Source: CAD feature listing. Evaluate the final solid. Frame: model axes, mm. A direction names the side the tool comes from. Round coordinates to 2 decimals unless told otherwise and drop trailing zeros. Loops run counter-clockwise (first coordinate to the right, second up) from the corner with the lowest first, then second, coordinate; pieces in that order, holes last. Notation, with made-up numbers: (72, 66) - (107, 66) arc R27 cw to (107, 91) - close; hole circle Ø1 at (53, 32.25). An arc over 180 degrees is marked (long way). Write item = value, one per line. Start each with the question number.
from build123d import *

# Parameters (mm, degrees)
SKETCH_W        = 40
SKETCH_H        = 40
PAD_DEPTH       = 5
SKETCH001_W     = 40
SKETCH001_H     = 5
PAD001_DEPTH    = 71
PAD002_DEPTH    = 40
SKETCH004_R     = 2.1
POCKET_DEPTH    = 10
SKETCH008_R     = 2.6
POCKET002_DEPTH = 30
SKETCH009_R     = 5
POCKET003_DEPTH = 5
FILLET_R        = 2
FILLET001_R     = 2
FILLET002_R     = 2
FILLET003_R     = 6


with BuildPart() as part:
    # Sketch → Pad (new body)
    with BuildSketch(Plane.XY):
        with Locations((20, 20)):
            Rectangle(SKETCH_W, SKETCH_H)
    extrude(amount=PAD_DEPTH)

    # Sketch001 (on DatumPlane) → Pad001 (join)
    with BuildSketch(Plane.XY.offset(5)):
        with Locations((20, -2.5)):
            Rectangle(SKETCH001_W, SKETCH001_H)
    extrude(amount=-PAD001_DEPTH)

    # Sketch002 (on DatumPlane) → Pad002 (join)
    with BuildSketch(Plane.YZ.offset(40)):
        Polygon((40, 0), (0, 0), (0, -16), align=None)
    extrude(amount=-PAD002_DEPTH)

    # Sketch004 → Pocket (cut)
    with BuildSketch(Plane(origin=(0, 0, 0), x_dir=(-1, 0, 0), z_dir=(0, 1, 0))):
        with Locations((-32, -61)):
            Circle(SKETCH004_R)
        with Locations((-32.0014529651, -34.0000000391)):
            Circle(SKETCH004_R)
    extrude(amount=-POCKET_DEPTH, mode=Mode.SUBTRACT)

    # Sketch008 → Pocket002 (cut)
    with BuildSketch(Plane.XY.offset(5)):
        with Locations((7, 10)):
            Circle(SKETCH008_R)
        with Locations((32, 10)):
            Circle(SKETCH008_R)
        with Locations((32, 30)):
            Circle(SKETCH008_R)
        with Locations((7, 30)):
            Circle(SKETCH008_R)
    extrude(amount=-POCKET002_DEPTH, mode=Mode.SUBTRACT)

    # Sketch009 (on DatumPlane) → Pocket003 (cut)
    with BuildSketch(Plane(origin=(0, 5.5172413793, -13.7931034483), x_dir=(1, 0, 0), z_dir=(0, 0.3713906764, -0.9284766909))):
        with Locations((7.014635, -4.727969)):
            Circle(SKETCH009_R)
        with Locations((31.764727, -4.731389)):
            Circle(SKETCH009_R)
        with Locations((31.809804, -26.362438)):
            Circle(SKETCH009_R)
        with Locations((6.861452, -26.34057)):
            Circle(SKETCH009_R)
    extrude(amount=-POCKET003_DEPTH, mode=Mode.SUBTRACT)

    # Fillet
    fillet_edges = [part.edges().sort_by_distance(p)[0] for p in [
        (40, 20, 5),
    ]]
    fillet(fillet_edges, radius=FILLET_R)

    # Fillet001
    fillet001_edges = [part.edges().sort_by_distance(p)[0] for p in [
        (19, 40, 5),
    ]]
    fillet(fillet001_edges, radius=FILLET001_R)

    # Fillet002
    fillet002_edges = [part.edges().sort_by_distance(p)[0] for p in [
        (0, 19, 5),
    ]]
    fillet(fillet002_edges, radius=FILLET002_R)

    # Fillet003
    fillet003_edges = [part.edges().sort_by_distance(p)[0] for p in [
        (40, -2.5, -66),
        (0, -2.5, -66),
    ]]
    fillet(fillet003_edges, radius=FILLET003_R)


solid = part.part
(1) Cut plane A-A (x = 31.5). State how many separate pieces and enclosed holes the cut face has, and give its area (3 significant figures).
(2) Cut plane B-B (z = -34). Output: boundary loops of the cut face in (x, y), and give its area (3 significant figures).
(3) Access query for faces 1 (the face through (31.74, 27.04, 0.2)), 2 (the face through (38.289, -2.465, -64.196)). Directions: +Z, -Z, +X, -X, +Y, -Y. A direction counts if a zero-diameter tool reaches every point of the face in a straight line with its end or side. Return the directions, or none.
(4) Pin query (flat end, axial travel): P1, Ø3, axis at x = 27, y = 21.5, coming from the -Z side; P2, Ø4, axis at x = 7, y = 10, coming from the -Z side; P3, Ø7, axis at x = 32, y = 30, coming from the -Z side; P4, Ø5, axis at x = 32, z = -61, coming from the +Y side. Return the tip coordinate at first contact, or that it passes through.
(5) Material intervals for line 1 along X through (y, z) = (10, -4); line 2 along X through (y, z) = (-3.6, -34); line 3 along Y through (x, z) = (32, 2.85), sorted ascending. Write a range as from..to.
(6) Mould query, pull axis Y, two halves, no side actions, for faces 3 (the face through (6.44, 27.46, 3.22)), 4 (the face through (20, 17, 5)), 5 (the face through (0.6, 39.43, 1.5)). Classes: +Y half, -Y half, draft (parallel to the pull), parting line (faces both ways), or undercut.
(7) Cut plane D-D (x = 7). Output: boundary loops of the cut face in (y, z), and give its area (3 significant figures).
(8) Cut plane C-C (x = 23). Output: boundary loops of the cut face in (y, z).
Solution:
q1.separate_pieces = 5
q1.enclosed_holes = 0
q1.area = 656 mm^2
q2.outline = (0, -5) - (29.9, -5) - (29.9, 0) - (0, 0) - close; (34.1, -5) - (40, -5) - (40, 0) - (34.1, 0) - close
q2.area = 179 mm^2
q3.face_1 = none
q3.face_2 = -Z, +X, +Y, -Y
q4.P1 = -8
q4.P2 = through
q4.P3 = -0.01
q4.P4 = 0
q5.line_1 = 0..4.4, 9.6..29.4, 34.6..40
q5.line_2 = 0..29.9, 34.1..40
q5.line_3 = -5..7.4, 12.6..27.4, 32.6..40
q6.face_3 = undercut
q6.face_4 = draft
q6.face_5 = +Y half
q7.outline = (-5, -66) - (0, -66) - (0, -16) - (5.26, -13.89) - (3.41, -9.25) - (7.4, -7.65) - (7.4, 5) - (-5, 5) - close; (12.6, -5.57) - (12.69, -5.54) - (14.55, -10.18) - (25.33, -5.87) - (23.48, -1.22) - (27.4, 0.35) - (27.4, 5) - (12.6, 5) - close; (32.6, 2.43) - (32.76, 2.49) - (34.61, -2.15) - (40, 0) - (40, 3) arc R2 ccw to (38, 5) - (32.6, 5) - close
q7.area = 695 mm^2
q8.outline = (-5, -66) - (0, -66) - (0, -16) - (40, 0) - (40, 3) arc R2 ccw to (38, 5) - (-5, 5) - close
